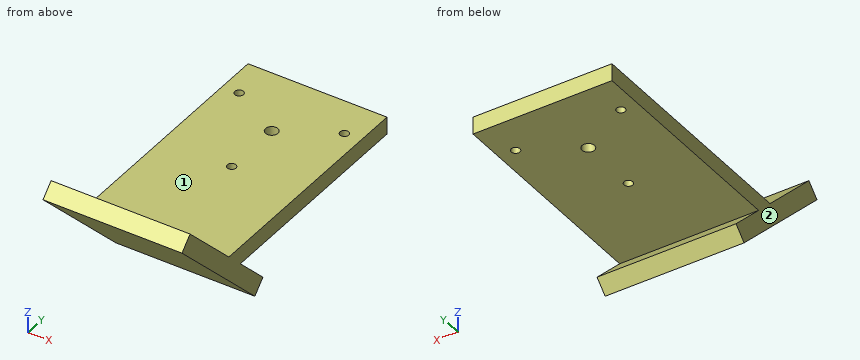
```python
from build123d import *

# Parameters (mm, degrees)
BOSS_EXTRUDE1_DEPTH   = 20
M3X0_5_TAPPED_HOLE1_D = 2.5
M3_CLEARANCE_HOLE1_D  = 3.6


with BuildPart() as part:
    # Sketch1 → Boss-Extrude1 (new, symmetric)
    with BuildSketch(Plane(origin=(0, 0, 0), x_dir=(0, 0, -1), z_dir=(1, 0, 0))):
        Polygon((-15.909902577, -15.909902577), (15.909902577, 15.909902577), (12.374368671, 19.445436483), (2.5, 9.571067812), (2.5, 73.613363655), (-2.5, 73.613363655), (-2.5, 4.571067812), (-19.445436483, -12.374368671), align=None)
    extrude(amount=BOSS_EXTRUDE1_DEPTH, both=True)

    # M3x0.5 Tapped Hole1 (through all)
    with Locations(Plane.XY.offset(2.5)):
        with Locations((-15.155444566, 62.363363655), (15.155444566, 62.363363655), (0, 36.113363655)):
            Hole(M3X0_5_TAPPED_HOLE1_D / 2)

    # M3 Clearance Hole1 (through all)
    with Locations(Plane.XY.offset(2.5)):
        with Locations((0, 53.613363655)):
            Hole(M3_CLEARANCE_HOLE1_D / 2)


solid = part.part
```
Input: part model. Units: mm. Frame: model coordinates. Face numbers are marked on the shaded views. A direction names the side the tool comes from. Coordinates: 2 decimals unless noted, no trailing zeros. Loops run counter-clockwise (first coordinate to the right, second up) from the corner with the lowest first, then second, coordinate; pieces in that order, holes last. Notation, with made-up numbers: M 51.5,74.5 L 87.5,74.5 A10 cw 87.5,92.5 Z; hole C -3,46.25 d4. An arc over 180 degrees is marked long. Use a Markdown table: item, result. Add a question column.
1) Pin query (flat end, axial travel): P1, Ø12, axis at x = 6.5, y = 54, coming from the +Z side; P2, Ø3, axis at x = -9, z = 13, coming from the +Y side; P3, Ø8, axis at x = -15, y = 12.5, coming from the -Z side; P4, Ø20, axis at x = -2, y = 38.5, coming from the -Z side. Return the tip coordinate at first contact, or that it passes through.
2) Set-up query: the marked faces 1 and 2. Return all of +Z, -Z, +X, -X, +Y, -Y with unobstructed straight access to the full face (end or side cutting, diameter ignored); none if empty.
3) Section D-D, the plane z = -4. Return the cut outline in (x, y).
4) Line query: L1, parallel to Y at x = 0, z = -1; L2, parallel to Y at x = 0, z = -0.45; L3, parallel to Z at x = 16, y = 44.5. Output: solid intervals per line, ascending. Write a range as from..to.
5) Section B-B, the plane y = 47. Return the cut outline in (x, z), plus the area to 3 significant figures.
6) Section A-A, the plane x = 0. Return the cut outline in (y, z).
7) Section C-C, the plane x = 10. Return the cut outline in (y, z).
Answer below:
| question | item | result |
|---|---|---|
| 1 | P1 | z = 2.5 |
| 1 | P2 | y = -4.43 |
| 1 | P3 | z = -15.91 |
| 1 | P4 | z = -2.5 |
| 2 | face 1 | +Z, +X, -X, +Y |
| 2 | face 2 | +Z, -Z, -X, +Y, -Y |
| 3 | outline | M -20,4 L 20,4 L 20,11.07 L -20,11.07 Z |
| 4 | L1 | 1..34.86, 37.36..51.81, 55.41..73.61 |
| 4 | L2 | 0.45..34.86, 37.36..51.81, 55.41..73.61 |
| 4 | L3 | -2.5..2.5 |
| 5 | outline | M -20,-2.5 L 20,-2.5 L 20,2.5 L -20,2.5 Z |
| 5 | area | 200 mm2 |
| 6 | outline | M -15.91,15.91 L 15.91,-15.91 L 19.45,-12.37 L 9.57,-2.5 L 34.86,-2.5 L 34.86,2.5 L 4.57,2.5 L -12.37,19.45 Z; M 37.36,-2.5 L 51.81,-2.5 L 51.81,2.5 L 37.36,2.5 Z; M 55.41,-2.5 L 73.61,-2.5 L 73.61,2.5 L 55.41,2.5 Z |
| 7 | outline | M -15.91,15.91 L 15.91,-15.91 L 19.45,-12.37 L 9.57,-2.5 L 73.61,-2.5 L 73.61,2.5 L 4.57,2.5 L -12.37,19.45 Z |
